```python
from build123d import *

# Parameters (mm, degrees)
F0_W     = 220
F0_H     = 33.712024
F1_DEPTH = 87.8


with BuildPart() as f1:
    # F0 (on Top) → F1 (new body)
    with BuildSketch(Plane.XY):
        Rectangle(F0_W, F0_H)
        with BuildLine():
            Line((-98.752904, 11.31518), (-48.752904, 11.31518))
            ThreePointArc((-48.752904, 11.31518), (-45.21737, 9.850714), (-43.752904, 6.31518))
            Line((-43.752904, 6.31518), (-43.752904, -6.31518))
            ThreePointArc((-43.752904, -6.31518), (-45.21737, -9.850714), (-48.752904, -11.31518))
            Line((-48.752904, -11.31518), (-98.752904, -11.31518))
            ThreePointArc((-98.752904, -11.31518), (-102.288438, -9.850714), (-103.752904, -6.31518))
            Line((-103.752904, -6.31518), (-103.752904, 6.31518))
            ThreePointArc((-103.752904, 6.31518), (-102.288438, 9.850714), (-98.752904, 11.31518))
        make_face(mode=Mode.SUBTRACT)
        with BuildLine():
            ThreePointArc((98.752904, 11.31518), (102.288438, 9.850714), (103.752904, 6.31518))
            Line((103.752904, 6.31518), (103.752904, -6.31518))
            ThreePointArc((103.752904, -6.31518), (102.288438, -9.850714), (98.752904, -11.31518))
            Line((98.752904, -11.31518), (48.752904, -11.31518))
            ThreePointArc((48.752904, -11.31518), (45.21737, -9.850714), (43.752904, -6.31518))
            Line((43.752904, -6.31518), (43.752904, 6.31518))
            ThreePointArc((43.752904, 6.31518), (45.21737, 9.850714), (48.752904, 11.31518))
            Line((48.752904, 11.31518), (98.752904, 11.31518))
        make_face(mode=Mode.SUBTRACT)
    extrude(amount=F1_DEPTH)


solid = f1.part
```
Verification items for the finished model (mm, model axes). A direction names the side the tool comes from. Coordinates: 2 decimals unless noted, no trailing zeros. Write each loop counter-clockwise with the first axis right and the second up, starting at its lowest first coordinate (ties: lowest second). Pieces come first, ordered by that corner, then holes. Notation, with made-up numbers: (55, 32.25) - (63, 32.25) arc R24 cw to (63, 53.25) - close; hole circle Ø5 at (-9, 75). An arc over 180 degrees is marked (long way). One line per question, with ' | ' between items. Start each with the question number.
1. Section check D-D (y = -9). Enter the section's corners in (x, z).
2. Section check B-B (x = 95). Enter the section's corners in (y, z), plus the area to 3 significant figures.
3. Section check A-A (y = 3). Enter the section's corners in (x, z).
4. Section check C-C (z = 5). Enter the section's corners in (x, y), plus the area to 3 significant figures.
5. Draft check along X on faces 3 (the cylindrical face through (102.25, 9.89, 43.29)), 4 (the flat face through (-110, 0, 43)), 5 (the flat face through (43.753, 0, 43)), 6 (the flat face through (-2, 0, 87.8)). Enter one of: released by +X, released by -X, zero draft, split by the parting line, or undercut.
6. Material ranges on line 1 along X through (y, z) = (7, 9.5); line 2 along X through (y, z) = (-5, 56); line 3 along Y through (x, z) = (-82, 59), recorded low to high.
7. Access from +Z, -Z, +X, -X, +Y, -Y to the whole of each face (thin tool, end or side, straight path). Record for faces 1 (the flat face through (-2, 0, 0)), 2 (the flat face through (-73, -11.315, 43)).
Computed values:
1) outline: (-110, 0) - (-102.97, 0) - (-102.97, 87.8) - (-110, 87.8) - close; (-44.53, 0) - (44.53, 0) - (44.53, 87.8) - (-44.53, 87.8) - close; (102.97, 0) - (110, 0) - (110, 87.8) - (102.97, 87.8) - close
2) outline: (-16.86, 0) - (-11.32, 0) - (-11.32, 87.8) - (-16.86, 87.8) - close; (11.32, 0) - (16.86, 0) - (16.86, 87.8) - (11.32, 87.8) - close | area: 973 mm²
3) outline: (-110, 0) - (-103.75, 0) - (-103.75, 87.8) - (-110, 87.8) - close; (-43.75, 0) - (43.75, 0) - (43.75, 87.8) - (-43.75, 87.8) - close; (103.75, 0) - (110, 0) - (110, 87.8) - (103.75, 87.8) - close
4) outline: (-110, -16.86) - (110, -16.86) - (110, 16.86) - (-110, 16.86) - close; hole (-103.75, -6.32) arc R5 ccw to (-98.75, -11.32) - (-48.75, -11.32) arc R5 ccw to (-43.75, -6.32) - (-43.75, 6.32) arc R5 ccw to (-48.75, 11.32) - (-98.75, 11.32) arc R5 ccw to (-103.75, 6.32) - close; hole (43.75, -6.32) arc R5 ccw to (48.75, -11.32) - (98.75, -11.32) arc R5 ccw to (103.75, -6.32) - (103.75, 6.32) arc R5 ccw to (98.75, 11.32) - (48.75, 11.32) arc R5 ccw to (43.75, 6.32) - close | area: 4,740 mm²
5) face 3: undercut | face 4: released by -X | face 5: undercut | face 6: zero draft
6) line 1: -110 to -103.71, -43.8 to 43.8, 103.71 to 110 | line 2: -110 to -103.75, -43.75 to 43.75, 103.75 to 110 | line 3: -16.86 to -11.32, 11.32 to 16.86
7) face 1: -Z, +X, -X, +Y, -Y | face 2: +Z, -Z
